Part model, mm, in its own coordinate system. Face numbers are marked on the shaded views. A direction names the side the tool comes from. Coordinates: 2 decimals unless noted, no trailing zeros. Loops run counter-clockwise (first coordinate to the right, second up) from the corner with the lowest first, then second, coordinate; pieces in that order, holes last. Notation, with made-up numbers: (5.5, -8) - (57.5, -8) arc R9 cw to (57.5, -2) - close; hole circle Ø5 at (76.5, 42.25). An arc over 180 degrees is marked (long way). Use a Markdown table: item, result. Add a question column.
1) Pull direction Z, two halves, no side cores. Call the marked faces 4, 5, 6 and 7: +Z half, -Z half, draft (parallel to the pull), parting line (faces both ways), or undercut.
2) Probe probe 1 along Y at (x, z) = (0, 9) (3 decimals); probe 2 along X at (y, z) = (-8.5, 31); probe 3 along Y at (x, z) = (26, 29.5). List the from-to ranges inside material, lowest first. Write a range as [from, to].
3) Drop flat-ended pins along their axis: P1, Ø13.5, axis at x = 58.5, z = 25, coming from the -Y side; P2, Ø2, axis at y = 4.5, z = 13.5, coming from the -X side; P3, Ø15, axis at x = 0, y = 0, coming from the +Z side (3 decimals); P4, Ø1.5, axis at y = 6.5, z = 34, coming from the -X side. Give the stop position or say it passes through.
4) Band-saw the part on B-B (y = -6). Give the cut face in (x, z).
5) Band-saw the part on A-A (x = 47.5). Give the cut face in (y, z).
6) Tool access for the marked faces 1, 2 and 3: list every direction of +Z, -Z, +X, -X, +Y, -Y with a clear straight run to the whole face (end or side of a thin tool).
from build123d import *

# Parameters (mm, degrees)
F0_R     = 9.525
F1_DEPTH = 44.45
F3_DEPTH = 12.701
F4_R     = 6.34999
F5_R     = 9.525


# Not quite as in the source:
# - a fillet or chamfer is up to 0.001 mm smaller than in the source, because OpenCascade refuses the exact size


with BuildPart() as f1:
    # F0 (on Top) → F1 (new body)
    with BuildSketch(Plane.XY):
        with BuildLine():
            Line((88.9, 19.05), (0, 19.05))
            ThreePointArc((0, 19.05), (-13.4703841816, -13.4703841816), (19.05, 0))
            Line((19.05, 0), (19.05, 6.35))
            Line((19.05, 6.35), (88.9, 6.35))
            Line((88.9, 6.35), (88.9, 19.05))
        make_face()
        Circle(F0_R, mode=Mode.SUBTRACT)
    extrude(amount=F1_DEPTH)

    # F2 (on face) → F3 (cut, through all)
    with BuildSketch(Plane.XZ.offset(-6.35)):
        with BuildLine():
            Line((88.9, 30.099), (38.1, 30.099))
            ThreePointArc((38.1, 30.099), (30.226, 22.225), (38.1, 14.351))
            Line((38.1, 14.351), (88.9, 14.351))
            Line((88.9, 14.351), (88.9, 30.099))
        make_face()
    extrude(amount=-F3_DEPTH, mode=Mode.SUBTRACT)

    # F4 (radius 6.35 in the source; OpenCascade refuses exactly that, so slightly less here)
    f4_edges = [f1.edges().sort_by_distance(p)[0] for p in [
        (19.05, 6.35, 22.225),
    ]]
    fillet(f4_edges, radius=F4_R)

    # F5
    f5_edges = [f1.edges().sort_by_distance(p)[0] for p in [
        (88.9, 12.7, 0),
        (88.9, 12.7, 44.45),
    ]]
    fillet(f5_edges, radius=F5_R)


solid = f1.part
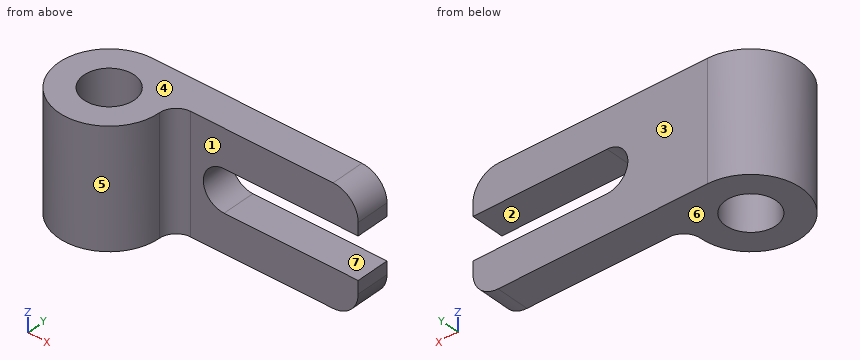
Answer block:
| question | item | result |
|---|---|---|
| 1 | face 4 | +Z half |
| 1 | face 5 | draft |
| 1 | face 6 | -Z half |
| 1 | face 7 | undercut |
| 2 | probe 1 | [-19.05, -9.525], [9.525, 19.05] |
| 2 | probe 2 | [-17.05, -4.3], [4.3, 17.05] |
| 2 | probe 3 | [6.35, 19.05] |
| 3 | P1 | y = 6.35 |
| 3 | P2 | x = -18.73 |
| 3 | P3 | through |
| 3 | P4 | x = -18.16 |
| 4 | outline | (-18.08, 0) - (-7.4, 0) - (-7.4, 44.45) - (-18.08, 44.45) - close; (7.4, 0) - (18.08, 0) - (18.08, 44.45) - (7.4, 44.45) - close |
| 5 | outline | (6.35, 0) - (19.05, 0) - (19.05, 14.35) - (6.35, 14.35) - close; (6.35, 30.1) - (19.05, 30.1) - (19.05, 44.45) - (6.35, 44.45) - close |
| 6 | face 1 | +Z, -Z, +X, -Y |
| 6 | face 2 | +X, +Y, -Y |
| 6 | face 3 | +Z, -Z, +X, -X, +Y |
